from build123d import *

# Parameters (mm, degrees)
SKETCH001_R = 19
PAD_DEPTH   = 15


with BuildPart() as part:
    # Sketch → Revolution (revolve)
    with BuildSketch(Plane.YZ):
        with BuildLine():
            Line((0, 0), (0, 50))
            Line((0, 50), (-4.5, 50))
            Line((-4.5, 50), (-4.5, 16.287714))
            ThreePointArc((-19, 0), (-9.24271, 5.911764), (-4.5, 16.287714))
            Line((0, 0), (-19, 0))
        make_face()
    revolve(axis=Axis((0, 0, 0), (0, 0, 1)))

    # Sketch001 (on Face4 of Revolution) → Pad (new body)
    with BuildSketch(Plane.YX):
        Circle(SKETCH001_R)
        Polygon((0, 13.914141), (-12.05, 6.957071), (-12.05, -6.957071), (0, -13.914141), (12.05, -6.957071), (12.05, 6.957071), align=None, mode=Mode.SUBTRACT)
    extrude(amount=PAD_DEPTH)


solid = part.part
The model under review builds one solid part; all positions refer to its coordinate system, in mm. A direction names the side the tool comes from. Coordinates: 2 decimals unless noted, no trailing zeros. Write each loop counter-clockwise with the first axis right and the second up, starting at its lowest first coordinate (ties: lowest second). Pieces come first, ordered by that corner, then holes. Notation, with made-up numbers: (60.5, 28) -> (76.5, 28) arc R26 cw to (76.5, 67) -> close; hole circle Ø3 at (72.25, 49). An arc over 180 degrees is marked (long way). Answer in a Markdown table with one row per item.
1. Clearance check with flat-ended pins moving along their axes: pin 1 Ø3 at (y, z) = (-1, -4.5) entering from -X; pin 2 Ø5 at (x, z) = (0.5, 36.5) entering from +Y; pin 3 Ø12 at (y, z) = (-4.5, 13) entering from -X. State where each tip first meets the part, or that it passes through.
Answers below:
| item | result |
|---|---|
| pin 1 | stops at x = -19 |
| pin 2 | stops at y = 4.5 |
| pin 3 | stops at x = -7.69 |
2. For faces 4 (the cylindrical face through (-16.856, 8.767, -7.395)), 5 (the flat face through (0, 0, 0)), list the 3-axis set-ups (+Z, -Z, +X, -X, +Y, -Y) from which the entire face can be reached by the end or side of a thin tool; tool diameter is ignored.
Answers below:
| item | result |
|---|---|
| face 4 | +Z, -Z |
| face 5 | -Z |
3. We need section B-B, the plane z = 30. State the section outline as (x, y) points, and give its area (3 significant figures).
Answers below:
| item | result |
|---|---|
| outline | circle Ø9 at (0, 0) |
| area | 63.6 mm^2 |
4. Wall thickness on probe 1 along X at (y, z) = (-8.5, 5.5); probe 2 along Z at (x, y) = (-2, -3); probe 3 along Y at (x, z) = (12.5, -3): over which ranges is each line inside the solid? List them lowest first. Write a range as [from, to].
Answers below:
| item | result |
|---|---|
| probe 1 | x = [-4.51, 4.51] |
| probe 2 | z = [0, 50] |
| probe 3 | y = [-14.31, -2.45], [2.45, 14.31] |
5. Draft analysis for pull direction X (two halves, no side actions). For faces 1 (the flat face through (0.3, 12.4, -15)), 2 (the flat face through (0, -12.05, -7)), 3 (the cylindrical face through (4.46, 0.59, 32.91)), state which applies: +X half, -X half, draft (parallel to the pull), parting line (faces both ways), or undercut.
Answers below:
| item | result |
|---|---|
| face 1 | draft |
| face 2 | undercut |
| face 3 | parting line |
6. We need section A-A, the plane x = 0. State the section outline as (y, z) points.
Answers below:
| item | result |
|---|---|
| outline | (-19, -15) -> (-12.05, -15) -> (-12.05, 0) -> (12.05, 0) -> (12.05, -15) -> (19, -15) -> (19, 0) arc R19.39 cw to (4.5, 16.29) -> (4.5, 50) -> (-4.5, 50) -> (-4.5, 16.29) arc R19.39 cw to (-19, 0) -> close |
7. We need section C-C, the plane z = 12. State the section outline as (x, y) points.
Answers below:
| item | result |
|---|---|
| outline | circle Ø11.14 at (0, 0) |
